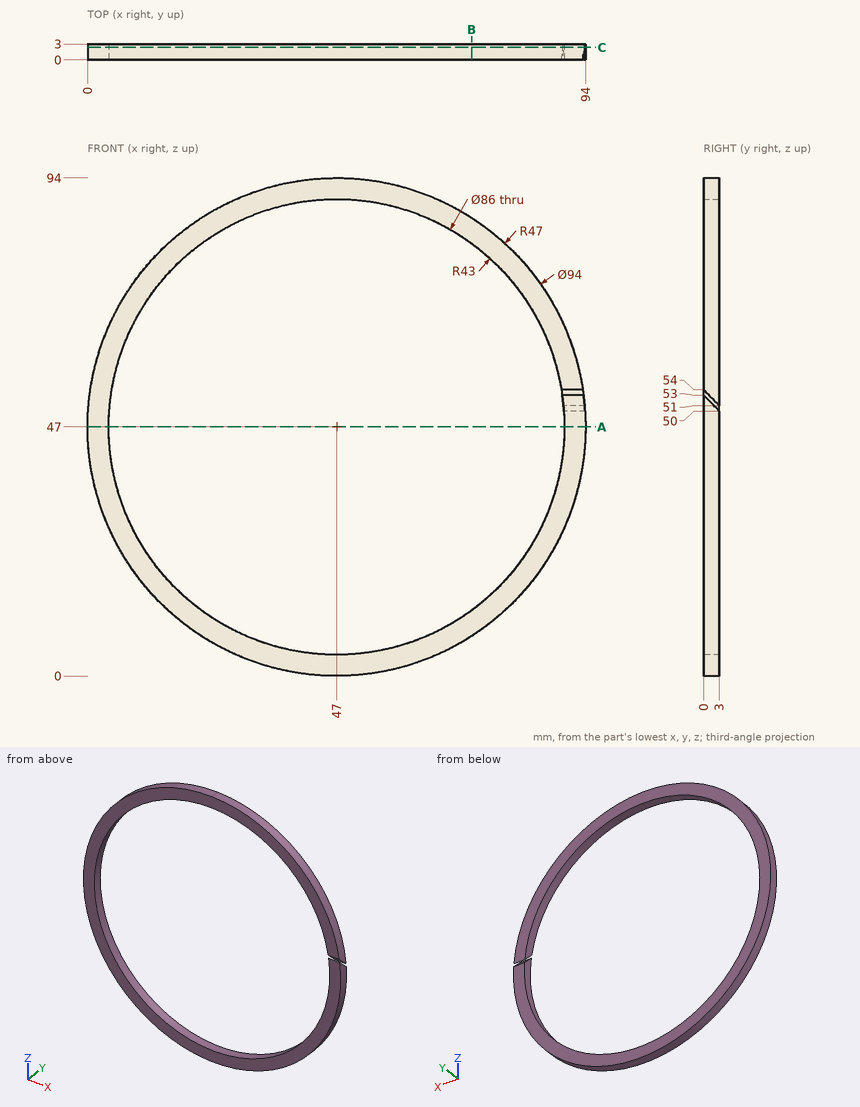
Answer from the drawing. Dimensions are ordinates in mm from the lowest x, y and z of the part. Coordinates: 2 decimals unless noted, no trailing zeros. Order: outer loops, then holes, each group sorted by start corner. A loop starts at its lowest first (then second) coordinate and runs counter-clockwise, first axis right, second up. Notation, with made-up numbers: (-21.75, 85.5) - (34.25, 85.5) arc R11 cw to (34.25, 103.5) - close; hole circle Ø10 at (-13, 65). An arc over 180 degrees is marked (long way). Answer as a JSON object with one key per item and string values. Group by question number.
Item 1: Consider probe 1 along Z at (x, y) = (47, 0.75); probe 2 along X at (y, z) = (2.3, 30). Determine where each line is inside the solid, lowest interval first. Write a range as from..to.
Item 2: Section B-B (x = 72.5) is taken. Give the vertices of the cut face in (y, z), plus the area to 3 significant figures.
Item 3: Section A-A (z = 47) is taken. Give the vertices of the cut face in (x, y).
Item 4: Section C-C (y = 2.35) is taken. Give the vertices of the cut face in (x, z).
Results are:
{
 "1": {"probe 1": "z = 0..4, 90..94", "probe 2": "x = 3.18..7.5, 86.5..90.82"},
 "2": {"outline": "(0, 7.52) - (3, 7.52) - (3, 12.38) - (0, 12.38) - close; (0, 81.62) - (3, 81.62) - (3, 86.48) - (0, 86.48) - close", "area": "29.1 mm^2"},
 "3": {"outline": "(0, 0) - (4, 0) - (4, 3) - (0, 3) - close; (90, 0) - (94, 0) - (94, 3) - (90, 3) - close"},
 "4": {"outline": "(89.75, 51.65) - (93.77, 51.65) arc R47 ccw (long way) to (93.86, 50.65) - (89.84, 50.65) arc R43 cw (long way) to start"}
}
